Print and shaded views of the part. All mm, measured from the part's lowest x, y and z. A direction names the side the tool comes from. Round coordinates to 2 decimals unless told otherwise and drop trailing zeros. Write each loop counter-clockwise with the first axis right and the second up, starting at its lowest first coordinate (ties: lowest second). Pieces come first, ordered by that corner, then holes. Notation, with made-up numbers: M 16.5,-37.75 L 59.5,-37.75 A14 ccw 59.5,-26.75 Z; hole C -27,84 d3. An arc over 180 degrees is marked long. Write item = value, one per line.
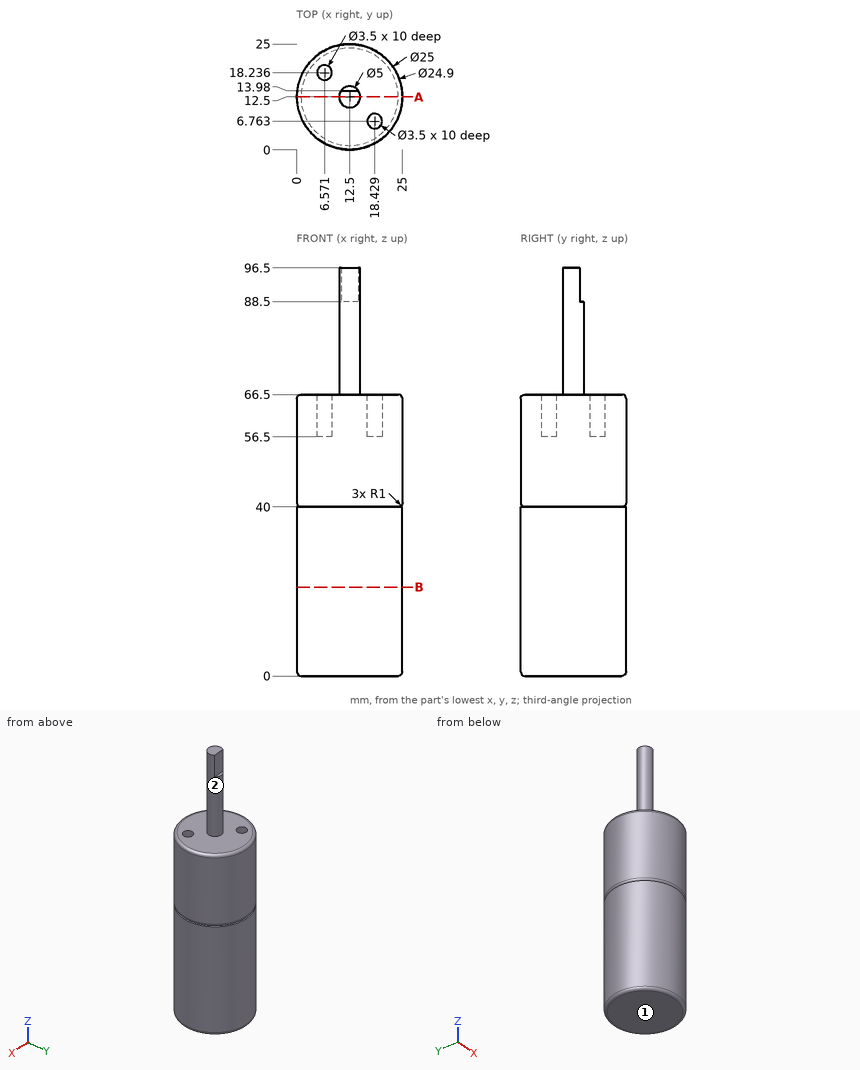
1. Band-saw the part on A-A (y = 12.5). List the corners of the cut face in (x, z).
Responses:
outline = M 0,41 A1 ccw 1,40 L 0.05,40 L 0.05,1 A1 ccw 1.05,0 L 23.95,0 A1 ccw 24.95,1 L 24.95,40 L 24,40 A1 ccw 25,41 L 25,65.5 A1 ccw 24,66.5 L 15,66.5 L 15,96.5 L 10,96.5 L 10,66.5 L 1,66.5 A1 ccw 0,65.5 Z
2. Flat gauge pins, fed straight in: pin 1 (6 mm diameter, centred on y = 9, z = 73.5, fed in from +X); pin 2 (5 mm diameter, centred on x = 20, y = 14, fed in from +Z); pin 3 (8 mm diameter, centred on y = 6.5, z = 28, fed in from -X). Where does each tip first touch, or does it go through?
Responses:
pin_1 = 14.95
pin_2 = 66.5
pin_3 = 0.21
3. Tool access for the marked faces 1 and 2: list every direction of +Z, -Z, +X, -X, +Y, -Y with a clear straight run to the whole face (end or side of a thin tool).
Responses:
face_1 = -Z, +X, -X, +Y, -Y
face_2 = +Z
4. Band-saw the part on B-B (z = 21). List the corners of the cut face in (x, y), plus the area to 3 significant figures.
Responses:
outline = C 12.5,12.5 d24.9
area = 487 mm²
5. Probe probe 1 along Y at (x, z) = (12.5, 43); probe 2 along Z at (x, y) = (18, 19.75); probe 3 along Y at (x, z) = (12.25, 4.5). List the from-to ranges inside material, lowest first.
Responses:
probe_1 = 0 to 25
probe_2 = 0 to 66.5
probe_3 = 0.05 to 24.95
